```python
from build123d import *

# Parameters (mm, degrees)
BOSS_EXTRUDE1_DEPTH = 0.6096
SKETCH5_R           = 2.25
CUT_EXTRUDE2_DEPTH  = 0.6096
SKETCH6_R           = 1.5875
CUT_EXTRUDE5_DEPTH  = 0.6096
SKETCH7_R           = 1.5875
CUT_EXTRUDE6_DEPTH  = 0.6096


with BuildPart() as part:
    # Sketch1 → Boss-Extrude1 (new body)
    with BuildSketch(Plane(origin=(16.997226787, -4.149929847, 204.631375634), x_dir=(0.9965694099183702, 0.001959509651517015, -0.0827379691367708), z_dir=(-0.08276069418699705, 0.02020630066742909, -0.9963645783100802))):
        Polygon((-405.631572024, 283.216979703), (-385.692572024, 283.216979703), (-385.692572024, 323.856979703), (-405.014358213, 323.856979703), (-432.414358217, 323.856979703), (-445.097076418, 323.856979703), (-465.359895626, 323.856979703), (-479.498480719, 323.856979703), (-500.373572024, 323.856979703), (-520.312572024, 323.856979703), (-520.312572024, 283.216979703), (-500.373572024, 283.216979703), (-500.373572024, 250.003685703), (-479.037572024, 250.003685703), (-479.037572024, 283.216979703), (-426.967572024, 283.216979703), (-426.967572024, 250.003685703), (-405.631572024, 250.003685703), align=None)
    extrude(amount=BOSS_EXTRUDE1_DEPTH)

    # Sketch5 → Cut-Extrude2 (cut)
    with BuildSketch(Plane(origin=(16.946775868, -4.137612086, 204.023991787), x_dir=(-0.9965694494101686, -0.0016780440853138524, 0.08274368054637986), z_dir=(-0.08276069418699686, 0.020206300667429084, -0.9963645783100801))):
        with Locations(Location((452.956635294, -318.984510283, 0), (0, 0, 0.096164523))):
            Circle(SKETCH5_R)
    cut_extrude2 = extrude(amount=-CUT_EXTRUDE2_DEPTH, mode=Mode.SUBTRACT)

    # Mirror1: Cut-Extrude2 across plane
    add(cut_extrude2.mirror(Plane(origin=(0.085159645, -303.474424262, -6.16154314), x_dir=(5.696257509048789e-06, -0.02029915071256956, 0.9997939509958544), z_dir=(0.00028055772663953236, -0.9997939116314238, -0.020299151511798782))), mode=Mode.SUBTRACT)

    # Sketch6 → Cut-Extrude5 (cut)
    with BuildSketch(Plane(origin=(16.946775868, -4.137612086, 204.023991787), x_dir=(-0.9965694494101686, -0.0016780440853136297, 0.08274368054637984), z_dir=(-0.08276069418699684, 0.02020630066742912, -0.9963645783100802))):
        with Locations(Location((416.50680125, -256.173836565, 0), (0, 0, 0.096164523))):
            Circle(SKETCH6_R)
    extrude(amount=-CUT_EXTRUDE5_DEPTH, mode=Mode.SUBTRACT)

    # Sketch7 → Cut-Extrude6 (cut)
    with BuildSketch(Plane(origin=(16.946775868, -4.137612086, 204.023991787), x_dir=(-0.9965694494101686, -0.0016780440853141857, 0.08274368054637986), z_dir=(-0.08276069418699686, 0.020206300667429056, -0.9963645783100801))):
        with Locations(Location((489.681466673, -256.194436956, 0), (0, 0, 0.096164523))):
            Circle(SKETCH7_R)
    extrude(amount=-CUT_EXTRUDE6_DEPTH, mode=Mode.SUBTRACT)


solid = part.part
```
Can you work these out from the model? Positions are in its coordinate system, mm. Round coordinates to 2 decimals unless told otherwise and drop trailing zeros. Loops run counter-clockwise (first coordinate to the right, second up) from the corner with the lowest first, then second, coordinate; pieces in that order, holes last. Notation, with made-up numbers: M -1.75,-4 L 14.25,-4 A23 ccw 14.25,25 Z; hole C 69.25,59 d10. An arc over 180 degrees is marked long. Write item = value, one per line. Start each with the question number.
(1) I'm going to push flat-ended pins straight in: P1, Ø3, axis at y = -283.5, z = 239.5, coming from the +X side; P2, Ø2, axis at x = -426, y = -298, coming from the -Z side; P3, Ø4, axis at x = -472, y = -265, coming from the -Z side. Where does each tip first touch, or does it pass through?
(2) Suppose I cut it at B-B on x = -468. Write out the boundary of the cut face in (y, z).
(3) Suppose I cut it at A-A on y = -270.5. Write out the boundary of the cut face in (x, z), plus the area to 3 significant figures.
(4) Suppose I cut it at C-C on y = -312. Write out the boundary of the cut face in (x, z).
(5) I need wall thicknesses on line 1 along Z through (x, y) = (-463.5, -302); line 2 along Z through (x, y) = (-410, -296.5). Which ranges of each line are inside material? Lowest first, please.
Answer block:
q1.P1 = -460.32
q1.P2 = 234.77
q1.P3 = 239.18
q2.outline = M -328.89,238.33 L -328.88,237.72 L -255.04,239.22 L -255.06,239.83 Z
q3.outline = M -481.64,240.04 L -460.37,238.27 L -460.32,238.88 L -481.59,240.64 Z; M -408.48,233.96 L -387.22,232.19 L -387.17,232.8 L -408.43,234.57 Z
q3.area = 26.0 mm²
q4.outline = M -501.49,240.84 L -367.34,229.7 L -367.29,230.31 L -501.44,241.45 Z
q5.line_1 = 237.89 to 238.5
q5.line_2 = 233.56 to 234.17
